Job drawing, mm, ordinate dimensions from the low corner. One solid piece. A direction names the side the tool comes from. Give positions to 0.01 mm unless a question says otherwise; leave off trailing zeros. Write each loop counter-clockwise with the first axis right and the second up, starting at its lowest first coordinate (ties: lowest second). Pieces come first, ordered by that corner, then holes. Notation, with made-up numbers: (22.25, 74.5) -> (79.25, 74.5) arc R25 ccw to (79.25, 111.5) -> close; hole circle Ø3 at (44.5, 8). An arc over 180 degrees is marked (long way). One line per question, with ' | ' between items. Start each with the question number.
(1) Pull direction Y, two halves, no side cores. Call the marked faces 3, 4 and 5: released by +Y, released by -Y, zero draft, split by the parting line, or undercut.
(2) Pin check, flat tips, straight feed: P1, Ø5, axis at x = 7.5, y = 22, coming from the +Z side; P2, Ø5, axis at y = 8, z = 6, coming from the -X side; P3, Ø8, axis at y = 4.5, z = 12, coming from the +X side. Stop position of each tip, or through.
(3) Drill centre lines: probe 1 along Z at (x, y) = (13, 6); probe 2 along Y at (x, z) = (35, 10.25) (1 decimal); probe 3 along Y at (x, z) = (20.5, 9). Where is each one in solid material? Low to high. Write a range as from..to.
(4) Tool access for the marked faces 1 and 2: list every direction of +Z, -Z, +X, -X, +Y, -Y with a clear straight run to the whole face (end or side of a thin tool).
(5) Band-saw the part on A-A, the plane y = 19. Give the cut face in (x, z) (1 decimal), and give its area (3 significant figures).
(6) Band-saw the part on B-B, the plane x = 15. Give the cut face in (y, z) (1 decimal), and give its area (3 significant figures).
(7) Band-saw the part on D-D, the plane y = 10. Give the cut face in (x, z), and give its area (3 significant figures).
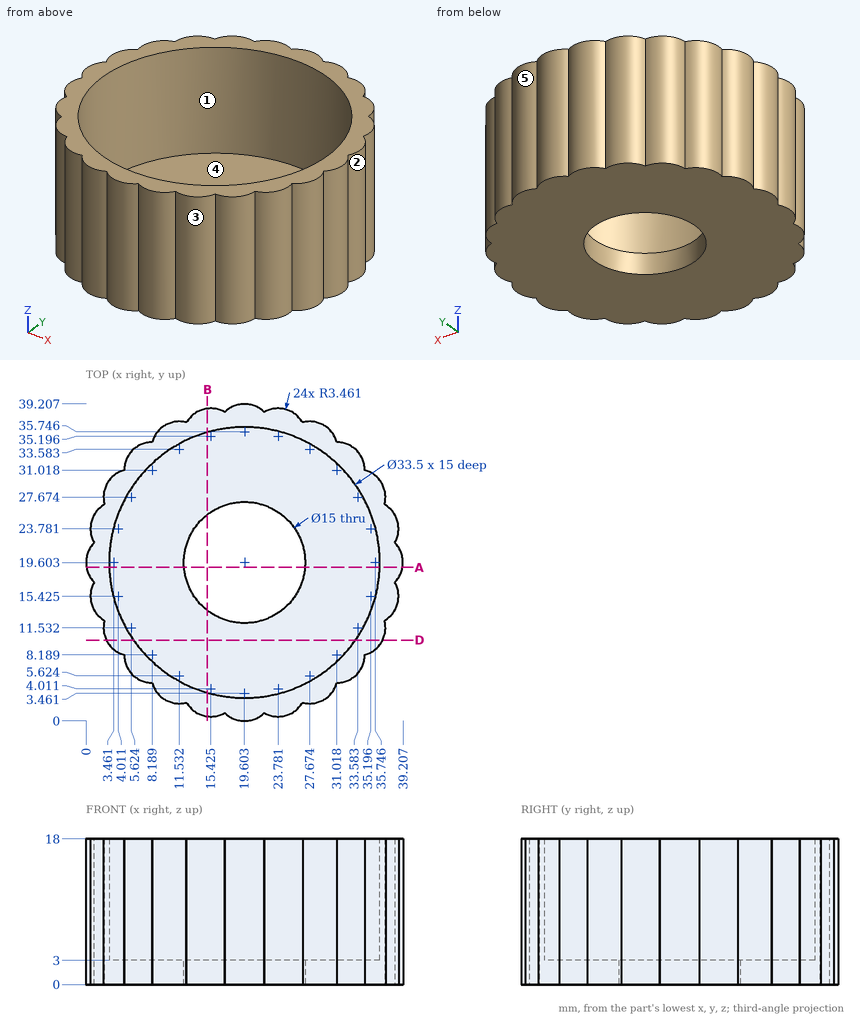
Results:
1) face 3: released by -Y | face 4: undercut | face 5: released by +Y
2) P1: stops at z = 3 | P2: stops at x = 2.32 | P3: stops at x = 35.25
3) probe 1: z = 0..3 | probe 2: y = 8.4..13, 26.2..30.8 | probe 3: y = 0.12..2.88, 36.33..39.09
4) face 1: +Z | face 2: +Z, -Z, +X
5) outline: (0.1, 0) -> (12.1, 0) -> (12.1, 3) -> (2.9, 3) -> (2.9, 18) -> (0.1, 18) -> close; (27.1, 0) -> (39.2, 0) -> (39.2, 18) -> (36.3, 18) -> (36.3, 3) -> (27.1, 3) -> close | area: 157 mm²
6) outline: (0.6, 0) -> (13.7, 0) -> (13.7, 3) -> (3.5, 3) -> (3.5, 18) -> (0.6, 18) -> close; (25.5, 0) -> (38.6, 0) -> (38.6, 18) -> (35.7, 18) -> (35.7, 3) -> (25.5, 3) -> close | area: 166 mm²
7) outline: (2.52, 0) -> (36.69, 0) -> (36.69, 18) -> (33.33, 18) -> (33.33, 3) -> (5.88, 3) -> (5.88, 18) -> (2.52, 18) -> close | area: 203 mm²
